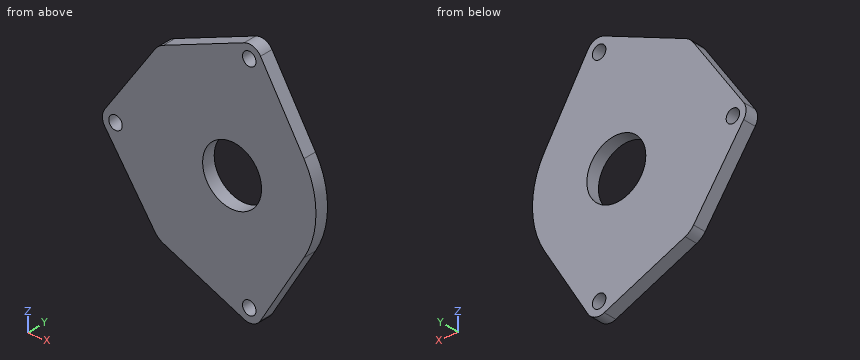
Autodesk Inventor part; units mm, degrees
ref_plane "YZ Plane" through (0, 0, 0) normal (1, 0, 0) x (0, 1, 0)
ref_plane "XZ Plane" through (0, 0, 0) normal (0, 1, 0) x (-1, 0, 0)
ref_plane "XY Plane" through (0, 0, 0) normal (0, 0, 1) x (1, 0, 0)
sketch "Sketch1" plane through (0, 0, 0) normal (0, 1, 0) x (-1, 0, 0)
  circle A0 centre (29.6155, 33.147) radius 6.35 construction
  circle A1 centre (0, 0) radius 38.1 construction
  circle A2 centre (29.6155, -33.147) radius 6.35 construction
  circle A3 centre (29.6155, 33.147) radius 29.972 construction
  circle A4 centre (29.6155, -33.147) radius 29.972 construction
  line L0 (29.6155, 3.175) -> (29.6155, -3.175) construction
  circle A5 centre (0, 0) radius 40.64 construction
  circle A6 centre (-8.3197, 52.6872) radius 6.35 construction
  circle A7 centre (-8.3197, 52.6872) radius 3.2639
  line L1 (-7.3293, 46.4149) -> (-6.3388, 40.1426) construction
  line L2 (-2.6746, 49.7794) -> (2.9705, 46.8716) construction
  circle A8 centre (-8.3197, -52.6872) radius 6.35 construction
  circle A9 centre (-8.3197, -52.6872) radius 3.2639
  line L3 (-7.3293, -46.4149) -> (-6.3388, -40.1426) construction
  line L4 (2.9705, -46.8716) -> (-2.6746, -49.7794) construction
  circle A10 centre (56.4888, 0) radius 6.35 construction
  circle A11 centre (56.4888, 0) radius 3.2639
  line L5 (48.4908, 9.8652) -> (52.4898, 4.9326) construction
  line L6 (52.4898, -4.9326) -> (48.4908, -9.8652) construction
  circle A12 centre (0, 0) radius 14.2875
  circle A13 centre (29.6155, 33.147) radius 9.525 construction
  circle A14 centre (29.6155, -33.147) radius 9.525 construction
  circle A15 centre (29.6155, 33.147) radius 25.4 construction
  circle A16 centre (29.6155, 58.547) radius 2.794 construction
  circle A17 centre (49.474, 48.9836) radius 2.794 construction
  circle A18 centre (54.3787, 27.495) radius 2.794 construction
  circle A19 centre (40.6362, 10.2624) radius 2.794 construction
  circle A20 centre (18.5949, 10.2624) radius 2.794 construction
  circle A21 centre (4.8523, 27.495) radius 2.794 construction
  circle A22 centre (9.757, 48.9836) radius 2.794 construction
  circle A23 centre (29.6155, -33.147) radius 25.4 construction
  circle A24 centre (29.6155, -58.547) radius 2.794 construction
  circle A25 centre (49.474, -48.9836) radius 2.794 construction
  circle A26 centre (54.3787, -27.495) radius 2.794 construction
  circle A27 centre (40.6362, -10.2624) radius 2.794 construction
  circle A28 centre (18.5949, -10.2624) radius 2.794 construction
  circle A29 centre (4.8523, -27.495) radius 2.794 construction
  circle A30 centre (9.757, -48.9836) radius 2.794 construction
  line L7 (37.4402, -38.5784) -> (61.7053, -3.6209)
  line L8 (61.7053, 3.6209) -> (37.4402, 38.5784)
  line L9 (33.335, 41.9157) -> (-5.84, 58.533)
  line L10 (-13.7609, 55.9607) -> (-34.8236, 20.9505)
  line L11 (-34.8236, -20.9505) -> (-13.7609, -55.9607)
  arc A31 (-34.8236, 20.9505) -> (-34.8236, -20.9505) centre (0, 0) ccw
  arc A32 (61.7053, -3.6209) -> (61.7053, 3.6209) centre (56.4888, 0) ccw
  arc A33 (37.4402, 38.5784) -> (33.335, 41.9157) centre (29.6155, 33.147) ccw
  arc A34 (-5.84, 58.533) -> (-13.7609, 55.9607) centre (-8.3197, 52.6872) ccw
  line L12 (-5.84, -58.533) -> (33.335, -41.9157)
  arc A35 (-13.7609, -55.9607) -> (-5.84, -58.533) centre (-8.3197, -52.6872) ccw
  arc A36 (33.335, -41.9157) -> (37.4402, -38.5784) centre (29.6155, -33.147) ccw
  point P0 (29.6155, 0)
  dimension "d21" = 50.8
  dimension "d27" = 50.8
  dimension "d0" = 12.7
  dimension "d1" = 76.2
  dimension "d2" = 12.7
  dimension "d3" = 59.944
  dimension "d4" = 59.944
  dimension "d5" = 6.35
  dimension "d6" = 2.54
  dimension "d8" = 12.7
  dimension "d9" = 6.5278
  dimension "d11" = 6.35
  dimension "d12" = 12.7
  dimension "d13" = 6.5278
  dimension "d14" = 6.35
  dimension "d15" = 12.7
  dimension "d16" = 6.5278
  dimension "d17" = 6.35
  dimension "d18" = 6.35
  dimension "d19" = 28.575
  dimension "d20" = 19.05
  dimension "d22" = 5.588
  dimension "d25" = 360
  dimension "d30" = 360
sketch "Sketch2" plane through (0, 0, 0) normal (0, 1, 0) x (-1, 0, 0)
  point P0 (0, 0)
extrude "Extrusion2" add sketch "Sketch1" along normal blind 6.35
properties part number "Bottom Plate" material "Aluminum 6061"
Here's how the part is built. I have some questions about the finished solid (model axes, mm). Coordinates: 2 decimals unless noted, no trailing zeros. Loops run counter-clockwise (first coordinate to the right, second up) from the corner with the lowest first, then second, coordinate; pieces in that order, holes last. Notation, with made-up numbers: (59.25, 22.5) -> (64.25, 22.5) arc R37 cw to (64.25, 60.5) -> close; hole circle Ø5 at (39, 86.25). An arc over 180 degrees is marked (long way). Return JSON: item names as keys, results as strings.
1) If we section it at B-B, the plane x = -56: Write out the boundary of the cut face in (y, z).
Results below:
{"outline": "(0, -11.84) -> (6.35, -11.84) -> (6.35, -3.23) -> (0, -3.23) -> close; (0, 3.23) -> (6.35, 3.23) -> (6.35, 11.84) -> (0, 11.84) -> close"}
2) If we section it at D-D, the plane x = 0: Write out the boundary of the cut face in (y, z).
Results below:
{"outline": "(0, -56.06) -> (6.35, -56.06) -> (6.35, -14.29) -> (0, -14.29) -> close; (0, 14.29) -> (6.35, 14.29) -> (6.35, 56.06) -> (0, 56.06) -> close"}
3) Will these pins go through, and if not, where does the flat tip stop? pin 1 (6 mm diameter, centred on x = -56.49, z = 0, fed in from -Y); pin 2 (2 mm diameter, centred on y = 1, z = 11, fed in from -X); pin 3 (2 mm diameter, centred on x = -12, y = 2.5, fed in from +Z); pin 4 (1 mm diameter, centred on y = 1.5, z = 37.5, fed in from +X).
Results below:
{"pin 1": "through", "pin 2": "x = -57.28", "pin 3": "z = 51.39", "pin 4": "x = 25.17"}
4) I need wall thicknesses on line 1 (Z direction, x = 0, y = 3.25); line 2 (Z direction, x = -55, y = 1.25); line 3 (X direction, y = 4, z = 26.5). Which ranges of each line are inside material? Lowest first, please. Write a range as from..to.
Results below:
{"line 1": "-56.06..-14.29, 14.29..56.06", "line 2": "-13.28..-2.9, 2.9..13.28", "line 3": "-45.82..31.48"}
5) If we section it at C-C, the plane y = 4: Write out the boundary of the cut face in (x, z) (1 decimal).
Results below:
{"outline": "(-61.7, -3.6) -> (-37.4, -38.6) arc R9.5 ccw to (-33.3, -41.9) -> (5.8, -58.5) arc R6.3 ccw to (13.8, -56) -> (34.8, -21) arc R40.6 ccw to (34.8, 21) -> (13.8, 56) arc R6.4 ccw to (5.8, 58.5) -> (-33.3, 41.9) arc R9.5 ccw to (-37.4, 38.6) -> (-61.7, 3.6) arc R6.4 ccw to start; hole circle Ø6.5 at (-56.5, 0); hole circle Ø28.6 at (0, 0); hole circle Ø6.5 at (8.3, -52.7); hole circle Ø6.5 at (8.3, 52.7)"}
6) If we section it at A-A, the plane z = 0: Write out the boundary of the cut face in (x, y), then the cut area to 3 significant figures.
Results below:
{"outline": "(-62.84, 0) -> (-59.75, 0) -> (-59.75, 6.35) -> (-62.84, 6.35) -> close; (-53.22, 0) -> (-14.29, 0) -> (-14.29, 6.35) -> (-53.22, 6.35) -> close; (14.29, 0) -> (40.64, 0) -> (40.64, 6.35) -> (14.29, 6.35) -> close", "area": "434 mm²"}
